```python
from build123d import *

# Parameters (mm, degrees)
BOSS_EXTRUDE1_DEPTH     = 40
BOSS_EXTRUDE2_START     = -2
BOSS_EXTRUDE2_OUTLINE_R = 1.6
BOSS_EXTRUDE2_DEPTH     = 2
FILLET1_R               = 1
FILLET2_R               = 1
SKETCH3_W               = 1.2
SKETCH3_H               = 2
SKETCH3_W_2             = 23.413110463
SKETCH3_H_2             = 14
CUT_EXTRUDE1_DEPTH      = 3
CHAMFER1_SIZE           = 3


# Read off the part's stored shape, not the designer's step: Boss-Extrude2
with BuildPart() as part:
    # Sketch1 → Boss-Extrude1 (new body)
    with BuildSketch(Plane(origin=(0, 0, 0), x_dir=(1, 0, 0), z_dir=(0, 1, 0))):
        with BuildLine():
            ThreePointArc((7.904340014, 6.355), (8.672424609, 5.833407053), (9.582575695, 5.65))
            Line((9.582575695, 5.65), (14, 5.65))
            ThreePointArc((14, 5.65), (17.288046533, 4.288046533), (18.65, 1))
            Line((18.65, 1), (18.65, 0))
            Line((18.65, 0), (16.15, 0))
            Line((16.15, 0), (16.15, 1))
            ThreePointArc((16.15, 1), (15.52027958, 2.52027958), (14, 3.15))
            Line((14, 3.15), (9.582575695, 3.15))
            ThreePointArc((9.582575695, 3.15), (7.704178772, 3.528520938), (6.118982907, 4.605))
            ThreePointArc((6.118982907, 4.605), (4.43573369, 5.748065396), (2.441147266, 6.15))
            Line((2.441147266, 6.15), (-0.15, 6.15))
            Line((-0.15, 6.15), (-0.15, 0))
            Line((-0.15, 0), (-2.65, 0))
            Line((-2.65, 0), (-2.65, 8.65))
            Line((-2.65, 8.65), (2.441147266, 8.65))
            ThreePointArc((2.441147266, 8.65), (5.403979526, 8.05295151), (7.904340014, 6.355))
        make_face()
    extrude(amount=BOSS_EXTRUDE1_DEPTH)

    # Boss-Extrude2 outline → Boss-Extrude2 (add)
    # profile 1 of 2: a face of its own
    with BuildSketch(Plane.XY.offset(BOSS_EXTRUDE2_START)):
        with BuildLine():
            Line((-2.65, 40), (-9.642066198, 32.445298796))
            ThreePointArc((-9.642066198, 32.445298796), (-10.351972428, 31.313118747), (-10.6, 30))
            Line((-10.6, 30), (-10.6, 10))
            ThreePointArc((-10.6, 10), (-10.351972428, 8.686881253), (-9.642066198, 7.554701204))
            Line((-9.642066198, 7.554701204), (-2.65, 0))
            Line((-2.65, 0), (-2.65, 40))
        make_face()
        with Locations((-7, 10)):
            Circle(BOSS_EXTRUDE2_OUTLINE_R, mode=Mode.SUBTRACT)
        with Locations((-7, 30)):
            Circle(BOSS_EXTRUDE2_OUTLINE_R, mode=Mode.SUBTRACT)
    # profile 2 of 2: a face of its own
    with BuildSketch(Plane.XY.offset(BOSS_EXTRUDE2_START)):
        with BuildLine():
            Line((26.6, 10), (26.6, 30))
            ThreePointArc((26.6, 30), (26.351972428, 31.313118747), (25.642066198, 32.445298796))
            Line((25.642066198, 32.445298796), (18.65, 40))
            Line((18.65, 40), (16.15, 40))
            Line((16.15, 40), (16.15, 0))
            Line((16.15, 0), (18.65, 0))
            Line((18.65, 0), (25.642066198, 7.554701204))
            ThreePointArc((25.642066198, 7.554701204), (26.351972428, 8.686881253), (26.6, 10))
        make_face()
        with Locations((23, 30)):
            Circle(BOSS_EXTRUDE2_OUTLINE_R, mode=Mode.SUBTRACT)
        with Locations((23, 10)):
            Circle(BOSS_EXTRUDE2_OUTLINE_R, mode=Mode.SUBTRACT)
    extrude(amount=BOSS_EXTRUDE2_DEPTH)

    # Fillet1
    fillet1_edges = [part.edges().sort_by_distance(p)[0] for p in [
        (-2.65, 20, -2),
        (-2.65, 20, -8.65),
        (18.541200282, 20, -2),
    ]]
    fillet(fillet1_edges, radius=FILLET1_R)

    # Fillet2
    fillet2_edges = [part.edges().sort_by_distance(p)[0] for p in [
        (16.15, 0, -0.5),
        (15.52027958, 0, -2.52027958),
        (11.791287847, 0, -3.15),
        (7.704178772, 0, -3.528520938),
        (4.43573369, 0, -5.748065396),
        (1.145573633, 0, -6.15),
        (-0.15, 0, -3.075),
        (-0.15, 40, -3.075),
        (1.145573633, 40, -6.15),
        (4.43573369, 40, -5.748065396),
        (7.704178772, 40, -3.528520938),
        (11.791287847, 40, -3.15),
        (15.52027958, 40, -2.52027958),
        (16.15, 40, -0.5),
    ]]
    fillet(fillet2_edges, radius=FILLET2_R)

    # Sketch3 → Cut-Extrude1 (cut)
    with BuildSketch(Plane.ZY.offset(10.6)):
        with Locations((-0.6, 32.977751257)):
            Rectangle(SKETCH3_W, SKETCH3_H)
        with Locations((-12.906555232, 32.977751257)):
            Rectangle(SKETCH3_W_2, SKETCH3_H)
        with Locations((-0.6, 24.977751257)):
            Rectangle(SKETCH3_W, SKETCH3_H_2)
        Polygon((0, 15.977751257), (0, 17.977751257), (-1.2, 17.977751257), (-15.374287906, 17.977751257), (-15.374287906, 15.977751257), align=None)
    extrude(amount=-CUT_EXTRUDE1_DEPTH, mode=Mode.SUBTRACT)

    # Chamfer1
    chamfer1_edges = [part.edges().sort_by_distance(p)[0] for p in [
        (-10.6, 17.977751257, -1.6),
    ]]
    chamfer(chamfer1_edges, length=CHAMFER1_SIZE - 0.0001)  # a hair under: the kernel refuses the full size


solid = part.part
```
Verification items for the finished model (mm, model axes). A direction names the side the tool comes from. Coordinates: 2 decimals unless noted, no trailing zeros. Loops run counter-clockwise (first coordinate to the right, second up) from the corner with the lowest first, then second, coordinate; pieces in that order, holes last. Notation, with made-up numbers: (58, -1) - (94, -1) arc R21 cw to (94, 14) - close; hole circle Ø5 at (-35, 46). An arc over 180 degrees is marked (long way). Put each result on its own line as item: value.
Item 1: Section check C-C (x = 13). Enter the section's corners in (y, z), then the cut area to 3 significant figures.
Conclusion:
outline: (0, -5.65) - (40, -5.65) - (40, -4.15) arc R1 ccw to (39, -3.15) - (1, -3.15) arc R1 ccw to (0, -4.15) - close
area: 99.6 mm2
Item 2: Section check B-B (y = 14.5). Enter the section's corners in (x, z) (3 decimals), then the cut area to 3 significant figures.
Conclusion:
outline: (-10.6, -2) - (-3.65, -2) arc R1 cw to (-2.65, -3) - (-2.65, -7.65) arc R1 ccw to (-1.65, -8.65) - (2.441, -8.65) arc R7.65 ccw to (7.904, -6.355) arc R2.35 cw to (9.583, -5.65) - (14, -5.65) arc R4.65 ccw to (18.349, -2.646) arc R1 cw to (19.284, -2) - (26.6, -2) - (26.6, 0) - (16.15, 0) - (16.15, -1) arc R2.15 cw to (14, -3.15) - (9.583, -3.15) arc R4.85 ccw to (6.119, -4.605) arc R5.15 cw to (2.441, -6.15) - (-0.15, -6.15) - (-0.15, 0) - (-10.6, 0) - close
area: 107 mm2
Item 3: Draft check along X on faces 1 (the face through (-7.6, 22, -1)), 2 (the face through (-4, 20, 0)), 3 (the face through (1.019, 39.699, -6.435)). Enter one of: pulls with the +X half, pulls with the -X half, needs draft (parallel to the pull), parting line crosses it, or undercut.
Conclusion:
face 1: pulls with the -X half
face 2: needs draft
face 3: undercut
Item 4: Section check A-A (x = -7). Enter the section's corners in (y, z).
Conclusion:
outline: (4.7, -2) - (8.4, -2) - (8.4, 0) - (4.7, 0) - close; (11.6, -2) - (28.4, -2) - (28.4, 0) - (11.6, 0) - close; (31.6, -2) - (35.3, -2) - (35.3, 0) - (31.6, 0) - close
Item 5: Set-up check for faces 4 (the face through (-0.435, 39.699, -3.525)), 5 (the face through (-9, 15.978, -1)), 6 (the face through (7.729, 19.734, -3.518)), 7 (the face through (-0.451, 0.285, -3.525)), 8 (the face through (7, 0, -6)): record each of +Z, -Z, +X, -X, +Y, -Y from which the full face is reachable in a straight line by a thin tool's end or side.
Conclusion:
face 4: +Z, +Y
face 5: +Z, -Z, -X
face 6: +Z, +Y, -Y
face 7: +Z, -Y
face 8: +Z, -Z, +X, -X, -Y
Item 6: Gauge pin test, flat ends, axial feed: pin 1 Ø4 at (y, z) = (18, -5.5) entering from -X; pin 2 Ø3 at (y, z) = (5.5, -6.5) entering from +X; pin 3 Ø0.7 at (x, z) = (-8, -1) entering from -Y. Record the tip position at first contact, or that the pin passes through.
Conclusion:
pin 1: stops at x = -2.65
pin 2: stops at x = 16.37
pin 3: stops at y = 5.4
Item 7: Scan lines: line 1 along X through (y, z) = (10.5, -0.75); line 2 along Y through (x, z) = (23, -0.5); line 3 along X through (y, z) = (14.5, -0.5). Record each from-to range of solid material in increasing order.
Conclusion:
line 1: x = -10.6 to -8.52, -5.48 to -0.15, 16.15 to 21.48, 24.52 to 26.6
line 2: y = 4.7 to 8.4, 11.6 to 28.4, 31.6 to 35.3
line 3: x = -10.6 to -0.15, 16.15 to 26.6
Item 8: Section check D-D (x = 24). Enter the section's corners in (y, z).
Conclusion:
outline: (5.78, -2) - (8.75, -2) - (8.75, 0) - (5.78, 0) - close; (11.25, -2) - (28.75, -2) - (28.75, 0) - (11.25, 0) - close; (31.25, -2) - (34.22, -2) - (34.22, 0) - (31.25, 0) - close
